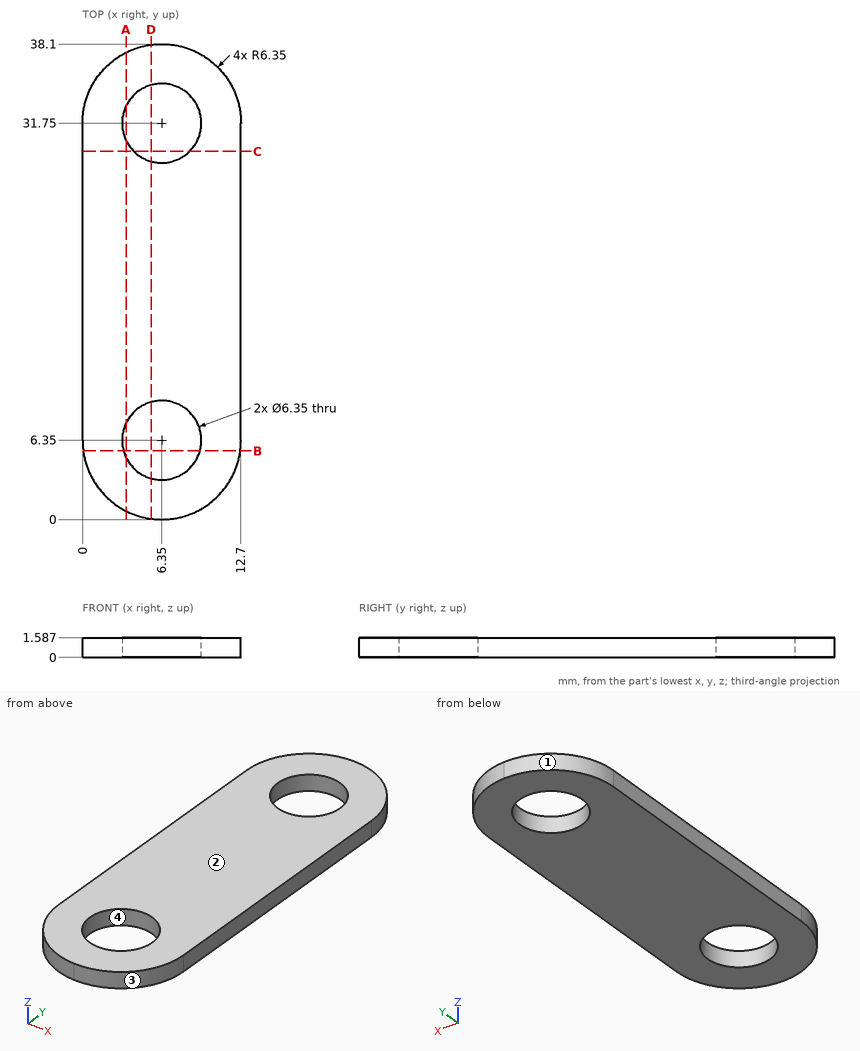
Study the drawing (mm; zero at the part's minimum x, y, z) and answer. Coordinates: 2 decimals unless noted, no trailing zeros. Write each loop counter-clockwise with the first axis right and the second up, starting at its lowest first coordinate (ties: lowest second). Pieces come first, ordered by that corner, then holes. Notation, with made-up numbers: (67, 58) - (79, 58) arc R11 cw to (79, 67) - close; hole circle Ø3 at (-3.5, 11). An arc over 180 degrees is marked (long way). Answer as a JSON object with one key per item and string values. Group by question number.
1. A cutting plane is placed at B-B (y = 5.5). Determine the outline of the cut face in (x, z).
2. Consider L1, parallel to Y at x = 6.35, z = 0.9 (1 decimal); L2, parallel to X at y = 6.5, z = 0.5; L3, parallel to Y at x = 8, z = 0.5. Determine where each line is inside the solid, lowest interval first. Write a range as [from, to].
3. A cutting plane is placed at D-D (x = 5.5). Determine the outline of the cut face in (y, z).
4. This flat-tipped pin is pushed along its axis until it touches: P1, Ø5, axis at x = 6.35, y = 31.75, coming from the +Z side. Where does it stop, or does it pass through?
5. A cutting plane is placed at C-C (y = 29.5). Determine the outline of the cut face in (x, z).
6. A cutting plane is placed at A-A (x = 3.5). Give the number of separate pieces and of enclosed holes in the cut face.
7. The mould has two halves that part along X. Classify the marked faces 1, 2, 3 and 4: +X half, -X half, draft (parallel to the pull), parting line (faces both ways), or undercut.
Worked out:
{
 "1": {"outline": "(0.06, 0) - (3.29, 0) - (3.29, 1.59) - (0.06, 1.59) - close; (9.41, 0) - (12.64, 0) - (12.64, 1.59) - (9.41, 1.59) - close"},
 "2": {"L1": "y = [0, 3.2], [9.5, 28.6], [34.9, 38.1]", "L2": "x = [0, 3.18], [9.52, 12.7]", "L3": "y = [0.22, 3.64], [9.06, 29.04], [34.46, 37.88]"},
 "3": {"outline": "(0.06, 0) - (3.29, 0) - (3.29, 1.59) - (0.06, 1.59) - close; (9.41, 0) - (28.69, 0) - (28.69, 1.59) - (9.41, 1.59) - close; (34.81, 0) - (38.04, 0) - (38.04, 1.59) - (34.81, 1.59) - close"},
 "4": {"P1": "passes through"},
 "5": {"outline": "(0, 0) - (4.11, 0) - (4.11, 1.59) - (0, 1.59) - close; (8.59, 0) - (12.7, 0) - (12.7, 1.59) - (8.59, 1.59) - close"},
 "6": {"separate pieces": "3", "enclosed holes": "0"},
 "7": {"face 1": "-X half", "face 2": "draft", "face 3": "+X half", "face 4": "undercut"}
}
